from build123d import *

# Parameters (mm, degrees)
SKETCH_1_R      = 22.071639064
SKETCH_1_R_2    = 2.6
EXTRUDE_1_DEPTH = 5


with BuildPart() as part:
    # 스케치1 → 보스-돌출1 (new body)
    with BuildSketch(Plane.XY):
        Circle(SKETCH_1_R)
        with Locations((0, 12.8)):
            Circle(SKETCH_1_R_2, mode=Mode.SUBTRACT)
        with Locations((-11.085125168, -6.4)):
            Circle(SKETCH_1_R_2, mode=Mode.SUBTRACT)
        with Locations((11.085125168, -6.4)):
            Circle(SKETCH_1_R_2, mode=Mode.SUBTRACT)
        with BuildLine():
            Line((-10, 5.5), (10, 5.5))
            Line((10, 5.5), (10, -1.5))
            Line((10, -1.5), (2.598076211, -1.5))
            ThreePointArc((2.598076211, -1.5), (0, -3), (-2.598076211, -1.5))
            Line((-2.598076211, -1.5), (-10, -1.5))
            Line((-10, -1.5), (-10, 5.5))
        make_face(mode=Mode.SUBTRACT)
    extrude(amount=EXTRUDE_1_DEPTH)


solid = part.part
Input: part model. Units: mm. Frame: model coordinates. A direction names the side the tool comes from. Give positions to 0.01 mm unless a question says otherwise; leave off trailing zeros. Order: outer loops, then holes, each group sorted by start corner. A loop starts at its lowest first (then second) coordinate and runs counter-clockwise, first axis right, second up.
Q1. Draft query along Y for faces 1 (the flat face through (0, -5, 5)), 2 (the cylindrical face through (-4.785, -21.547, 2.465)), 3 (the cylindrical face through (12.3, -8.7, 2.5)). Return one class per face: +Y half, -Y half, draft (parallel to the pull), parting line (faces both ways), or undercut.
Checked values:
face 1: draft
face 2: parting line
face 3: undercut
Q2. Section A-A on x = 0. Output: boundary loops of the cut face in (y, z), and give its area (3 significant figures).
Checked values:
outline: (-22.07, 0) - (-3, 0) - (-3, 5) - (-22.07, 5) - close; (5.5, 0) - (10.2, 0) - (10.2, 5) - (5.5, 5) - close; (15.4, 0) - (22.07, 0) - (22.07, 5) - (15.4, 5) - close
area: 152 mm2
Q3. Section B-B on y = 0. Output: boundary loops of the cut face in (x, z).
Checked values:
outline: (-22.07, 0) - (-10, 0) - (-10, 5) - (-22.07, 5) - close; (10, 0) - (22.07, 0) - (22.07, 5) - (10, 5) - close
Q4. Section D-D on x = 6. Output: boundary loops of the cut face in (y, z), and give its area (3 significant figures).
Checked values:
outline: (-21.24, 0) - (-1.5, 0) - (-1.5, 5) - (-21.24, 5) - close; (5.5, 0) - (21.24, 0) - (21.24, 5) - (5.5, 5) - close
area: 177 mm2
Q5. Section C-C on z = 0.55. Output: boundary loops of the cut face in (x, y).
Checked values:
outline: circle Ø44.14 at (0, 0); hole circle Ø5.2 at (-11.09, -6.4); hole (-10, -1.5) - (-2.6, -1.5) arc R3 ccw to (2.6, -1.5) - (10, -1.5) - (10, 5.5) - (-10, 5.5) - close; hole circle Ø5.2 at (0, 12.8); hole circle Ø5.2 at (11.09, -6.4)
Q6. Contact query for flat-ended pins moving along their axis: pin 1 Ø1 at (y, z) = (-10.5, 1) entering from -X; pin 2 Ø3 at (x, z) = (11, 0.5) entering from -Y; pin 3 Ø1.5 at (x, z) = (3.5, 3) entering from -Y. Output: stop coordinate, or through.
Checked values:
pin 1: stops at x = -19.68
pin 2: stops at y = -19.92
pin 3: stops at y = -21.9
Q7. Set-up query: faces 4 (the cylindrical face through (0, -3, 2)), 5 (the flat face through (0, -5, 0)). Return all of +Z, -Z, +X, -X, +Y, -Y with unobstructed straight access to the full face (end or side cutting, diameter ignored); none if empty.
Checked values:
face 4: +Z, -Z
face 5: -Z, +X, -X, +Y, -Y
Q8. Ray query, probe 1 along Y at (x, z) = (0, 3.6); probe 2 along Y at (x, z) = (-1, 3.8); probe 3 along Y at (x, z) = (-11.5, 1.2). Return the intervals inside material, ascending.
Checked values:
probe 1: y = -22.07 to -3, 5.5 to 10.2, 15.4 to 22.07
probe 2: y = -22.05 to -2.83, 5.5 to 10.4, 15.2 to 22.05
probe 3: y = -18.84 to -8.97, -3.83 to 18.84
